Source: CAD feature listing. Evaluate the final solid. Frame: model axes, mm. Coordinates: 2 decimals unless noted, no trailing zeros. Order: outer loops, then holes, each group sorted by start corner. A loop starts at its lowest first (then second) coordinate and runs counter-clockwise, first axis right, second up. Notation, with made-up numbers: (-17.5, 57) - (27.5, 57) arc R16 ccw to (27.5, 83) - close; hole circle Ø10 at (24, 16.25). An arc over 180 degrees is marked (long way). One line per question, with ' | ' between items. Start each with the question number.
(1) Line query: line 1 along Y through (x, z) = (0, 94); line 2 along Z through (x, y) = (17, 2.75); line 3 along Z through (x, y) = (-19.5, 5.75) (3 decimals). Output: solid intervals per line, ascending.
(2) Section B-B (z = -118). Return the cut outline in (x, y).
(3) Draft query along X for faces 1 (the flat face through (-1, 5, 96.445)), 2 (the flat face through (39.5, 3, 1)), 3 (the cylindrical face through (-35.293, 3.131, -98.676)), 4 (the cylindrical face through (-6.61, 3.13, -66.67)). Return one class per face: +X half, -X half, draft (parallel to the pull), parting line (faces both ways), or undercut.
(4) Contact query for flat-ended pins moving along their axis: P1, Ø4, axis at x = -17.5, z = -126.76, coming from the -Y side; P2, Ø2, axis at x = -9.5, y = 3.5, coming from the -Z side; P3, Ø1.8, axis at x = 0, y = 3.175, coming from the -Z side (3 decimals); P4, Ø1.8, axis at x = 17.25, y = 3.175, coming from the -Z side. Output: stop coordinate, or through.
(5) Section A-A (x = 22.5). Return the cut outline in (y, z) (3 decimals), then the cut area to 3 significant figures.
from build123d import *

# Parameters (mm, degrees)
BOSS_EXTRUDE1_OUTLINE_R      = 2.25
BOSS_EXTRUDE1_OUTLINE_R_2    = 30.5
BOSS_EXTRUDE1_DEPTH          = 6.35
M2_5X0_45_TAPPED_HOLE1_D     = 2.05
M2_5X0_45_TAPPED_HOLE1_DEPTH = 6.35
M2_5X0_45_TAPPED_HOLE1_TIP   = 0.615882135


# Read off the part's stored shape, not the designer's step: Boss-Extrude1
with BuildPart() as part:
    # Boss-Extrude1 outline → Boss-Extrude1 (new body)
    with BuildSketch(Plane(origin=(0, 0, 0), x_dir=(1, 0, 0), z_dir=(0, 1, 0))):
        with BuildLine():
            ThreePointArc((39.5, 96.444999522), (2.39e-07, 135.945), (-39.5, 96.445))
            Line((-39.5, 96.445), (-39.500001167, -96.445))
            Line((-39.500001167, -96.445), (39.499998833, -96.445000478))
            Line((39.499998833, -96.445000478), (39.5, 96.444999522))
        make_face()
        with Locations((-17.5, 66.134110868)):
            Circle(BOSS_EXTRUDE1_OUTLINE_R, mode=Mode.SUBTRACT)
        with Locations((-35, 96.445)):
            Circle(BOSS_EXTRUDE1_OUTLINE_R, mode=Mode.SUBTRACT)
        with Locations((-17.5, 126.755889132)):
            Circle(BOSS_EXTRUDE1_OUTLINE_R, mode=Mode.SUBTRACT)
        with Locations((17.5, 66.134110868)):
            Circle(BOSS_EXTRUDE1_OUTLINE_R, mode=Mode.SUBTRACT)
        with Locations((0, 96.445)):
            Circle(BOSS_EXTRUDE1_OUTLINE_R_2, mode=Mode.SUBTRACT)
        with Locations((17.5, 126.755889132)):
            Circle(BOSS_EXTRUDE1_OUTLINE_R, mode=Mode.SUBTRACT)
        with Locations((35, 96.445)):
            Circle(BOSS_EXTRUDE1_OUTLINE_R, mode=Mode.SUBTRACT)
    extrude(amount=BOSS_EXTRUDE1_DEPTH)

    # M2.5x0.45 Tapped Hole1
    with Locations(Plane(origin=(-5.84e-07, 0, 96.445000239), x_dir=(1.0, 0, 6.0503381489132905e-09), z_dir=(-6.0503381489132905e-09, 0, 1.0))):
        with Locations((0, 3.175), (17.249999708, 3.175), (34.499999416, 3.175), (-17.249999708, 3.175), (-34.499999416, 3.175)):
            Hole(M2_5X0_45_TAPPED_HOLE1_D / 2, depth=M2_5X0_45_TAPPED_HOLE1_DEPTH)
            with Locations((0, 0, -(M2_5X0_45_TAPPED_HOLE1_DEPTH + M2_5X0_45_TAPPED_HOLE1_TIP / 2))):  # 118° drill point
                Cone(0, M2_5X0_45_TAPPED_HOLE1_D / 2, M2_5X0_45_TAPPED_HOLE1_TIP, mode=Mode.SUBTRACT)


solid = part.part
Response values:
1) line 1: y = 0 to 2.15, 4.2 to 6.35 | line 2: z = -132.1 to -128.95, -124.56 to -121.77, -71.12 to -68.33, -63.94 to 89.78 | line 3: z = -130.796 to -127.787, -125.725 to -119.897, -72.993 to -67.165, -65.103 to 96.445
2) outline: (-33.1, 0) - (-21.58, 0) - (-21.58, 6.35) - (-33.1, 6.35) - close; (21.58, 0) - (33.1, 0) - (33.1, 6.35) - (21.58, 6.35) - close
3) face 1: draft | face 2: +X half | face 3: undercut | face 4: undercut
4) P1: passes through | P2: stops at z = -135.02 | P3: stops at z = -135.945 | P4: stops at z = -132.4
5) outline: (0, -128.91) - (6.35, -128.91) - (6.35, -117.036) - (0, -117.036) - close; (0, -75.854) - (6.35, -75.854) - (6.35, 96.445) - (0, 96.445) - close | area: 1,170 mm²
